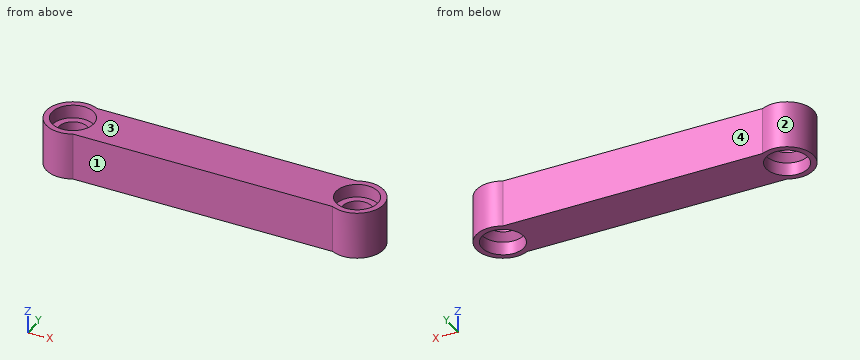
Autodesk Inventor part; units mm, degrees
ref_plane "YZ Plane" through (0, 0, 0) normal (1, 0, 0) x (0, 1, 0)
ref_plane "XZ Plane" through (0, 0, 0) normal (0, 1, 0) x (-1, 0, 0)
ref_plane "XY Plane" through (0, 0, 0) normal (0, 0, 1) x (1, 0, 0)
sketch "Sketch1" plane through (0, 0, 0) normal (0, 0, 1) x (1, 0, 0)
  line L0 (0, 12.5) -> (149.8, 12.5)
  arc A0 (149.8, -12.5) -> (149.8, 12.5) centre (149.8, 0) ccw
  line L1 (149.8, -12.5) -> (0, -12.5)
  arc A1 (0, 12.5) -> (0, -12.5) centre (0, 0) ccw
  dimension "d0" = 149.8
  dimension "d2" = 12.5
extrude "Extrusion1" add sketch "Sketch1" along normal blind 25
sketch "Sketch2" plane through (0, 0, 25) normal (0, 0, 1) x (1, 0, 0)
  arc A0 (0, 12.5) -> (0, -12.5) centre (0, 0) ccw
  arc A1 (149.8, -12.5) -> (149.8, 12.5) centre (149.8, 0) ccw
  circle A2 centre (0, 0) radius 7.55
  circle A3 centre (149.8, 0) radius 7.55
  dimension "d5" = 15.1
extrude "Extrusion2" cut sketch "Sketch2" against normal through all
sketch "Sketch3" plane through (0, 0, 25) normal (0, 0, 1) x (1, 0, 0)
  circle A0 centre (0, 0) radius 7.55
  circle A1 centre (149.8, 0) radius 7.55
  arc A2 (0, 12.5) -> (0, -12.5) centre (0, 0) ccw
  arc A3 (149.8, -12.5) -> (149.8, 12.5) centre (149.8, 0) ccw
  circle A4 centre (0, 0) radius 11.05
  circle A5 centre (149.8, 0) radius 11.05
  dimension "d9" = 22.1
extrude "Extrusion3" cut sketch "Sketch3" against normal blind 7
sketch "Sketch4" plane through (0, 0, 0) normal (0, 0, -1) x (-1, 0, 0)
  circle A0 centre (0, 0) radius 7.55
  circle A1 centre (-149.8, 0) radius 7.55
  circle A2 centre (-149.8, 0) radius 11.05
  circle A3 centre (0, 0) radius 11.05
extrude "Extrusion4" cut sketch "Sketch4" against normal blind 7
chamfer "Chamfer1" distance 3.5 angle 45 2 edges at (142.25, 0, 7) (-7.55, 0, 7)
sketch "Sketch5" plane through (0, 0, 25) normal (0, 0, 1) x (1, 0, 0)
  circle A0 centre (0, 0) radius 11.05
  circle A1 centre (149.8, 0) radius 11.05
  arc A2 (0, 12.5) -> (0, -12.5) centre (0, 0) ccw
  arc A3 (149.8, -12.5) -> (149.8, 12.5) centre (149.8, 0) ccw
  circle A4 centre (0, 0) radius 14.05
  circle A5 centre (149.8, 0) radius 14.05
  dimension "d18" = 3
extrude "Extrusion5" add sketch "Sketch5" against normal up to surface (25 mm away)
ref_plane "Work Plane2" through (6.8813, -12.5, 23) normal (0, -1, 0) x (1, 0, 0)
sketch "Sketch6" plane through (6.415, -12.5, 0) normal (0, -1, 0) x (1, 0, 0)
  line L0 (0, 0) -> (136.97, 2.0217)
  line L1 (136.97, 2.0217) -> (131.3954, 22.9783)
  line L2 (0, 25) -> (136.97, 25) construction
  line L3 (136.97, 25) -> (136.97, 0) construction
  line L4 (136.97, 0) -> (0, 0) construction
  line L5 (0, 0) -> (0, 25) construction
  line L6 (136.97, 0) -> (136.97, 25)
  line L7 (0, 25) -> (136.97, 25)
  point P0 (-6.8813, -23)
  point P1 (136.97, 12.5)
  point P2 (134.1827, 12.5)
  point P3 (68.485, 25)
  point P4 (68.485, 1.0109)
ref_plane "Work Plane1" through (6.8813, 12.5, 23) normal (0, 1, 0) x (1, 0, 0)
sketch "Sketch7" plane through (6.8813, 12.5, 23) normal (0, 1, 0) x (1, 0, 0)
  line L0 (136.5037, 23) -> (-0.4663, 23) construction
  line L1 (-0.4663, 23) -> (-0.4663, -2) construction
  line L2 (-0.4663, -2) -> (136.5037, -2) construction
  line L3 (136.5037, -2) -> (136.5037, 23) construction
  line L4 (136.5037, -2) -> (136.5037, 23)
  line L5 (-0.4663, 23) -> (136.5037, 23)
  line L6 (-0.4663, 23) -> (-0.4663, -2)
  line L7 (136.5037, -2) -> (-0.4663, -2)
  point P0 (-6.8813, 23)
extrude "Extrusion6" [suppressed]
extrude "Extrusion7" [suppressed]
properties part number "xy wall arm SP"
Could you check a few things on this model? Use its own coordinates, in mm. Face numbers are marked on the shaded views. A direction names the side the tool comes from. Round coordinates to 2 decimals unless told otherwise and drop trailing zeros. Loops run counter-clockwise (first coordinate to the right, second up) from the corner with the lowest first, then second, coordinate; pieces in that order, holes last. Notation, with made-up numbers: M -6.75,4 L 47.25,4 A25 cw 47.25,24 Z; hole C 42,-23 d11. An arc over 180 degrees is marked long. Answer as CSV lines item,"result".
1) If I drill on probe 1 along X at (y, z) = (0, 4.75); probe 2 along Y at (x, z) = (0, 15.25); probe 3 along Y at (x, z) = (149.8, 2.25), over which ranges is the centre line in solid material (lowest first)?
From the geometry:
probe 1,"-14.05 to -11.05, 11.05 to 138.75, 160.85 to 163.85"
probe 2,"-14.05 to -7.55, 7.55 to 14.05"
probe 3,"-14.05 to -11.05, 11.05 to 14.05"
2) Imagine slicing it at C-C on y = -4.75. Count the separate pieces of the cut face and the enclosed holes in it, and give its area (3 significant figures).
From the geometry:
separate pieces,"3"
enclosed holes,"0"
area,"3,560 mm^2"
3) Imagine slicing it at D-D on x = 26. List the corners of the cut face in (y, z) for me.
From the geometry:
outline,"M -12.5,0 L 12.5,0 L 12.5,25 L -12.5,25 Z"
4) Imagine slicing it at B-B on z = 12.5. List the corners of the cut face in (x, y) for me, and give its area (3 significant figures).
From the geometry:
outline,"M 6.42,-12.5 L 143.38,-12.5 A14.05 ccw long 143.38,12.5 L 6.42,12.5 A14.05 ccw long Z; hole C 0,0 d15.1; hole C 149.8,0 d15.1"
area,"4,030 mm^2"
5) Which directions (+Z, -Z, +X, -X, +Y, -Y) give clear straight access to the entire face, cutting with the end or side of a thin tool? Please do the marked faces 1 and 2.
From the geometry:
face 1,"+Z, -Z, -Y"
face 2,"+Z, -Z"
6) We'd pull the mould along X, two halves only. Please class the marked faces 3 and 4: released by +X, released by -X, zero draft, split by the parting line, or undercut.
From the geometry:
face 3,"zero draft"
face 4,"undercut"
7) For pin 1 Ø1 at (x, z) = (91, 10.5) entering from +Y; pin 2 Ø2 at (x, y) = (87.5, 8.5) entering from -Z; pin 3 Ø12 at (y, z) = (-10.5, 13.5) entering from +X; pin 4 Ø6.5 at (x, y) = (151.5, -5) entering from +Z, each with a flat end and sliding along its axis, tell me the tip position at first contact or that it passes through.
From the geometry:
pin 1,"y = 12.5"
pin 2,"z = 0"
pin 3,"x = 163.11"
pin 4,"z = 18"
